Here's how the part is built. I have some questions about the finished solid (model axes, mm). Face numbers are marked on the shaded views. A direction names the side the tool comes from. Give positions to 0.01 mm unless a question says otherwise; leave off trailing zeros. Loops run counter-clockwise (first coordinate to the right, second up) from the corner with the lowest first, then second, coordinate; pieces in that order, holes last. Notation, with made-up numbers: (82.25, 9) - (98.25, 9) arc R20 ccw to (98.25, 36) - close; hole circle Ø11 at (66.25, 29). An arc over 180 degrees is marked (long way). Put each result on its own line as item: value. Start each with the question number.
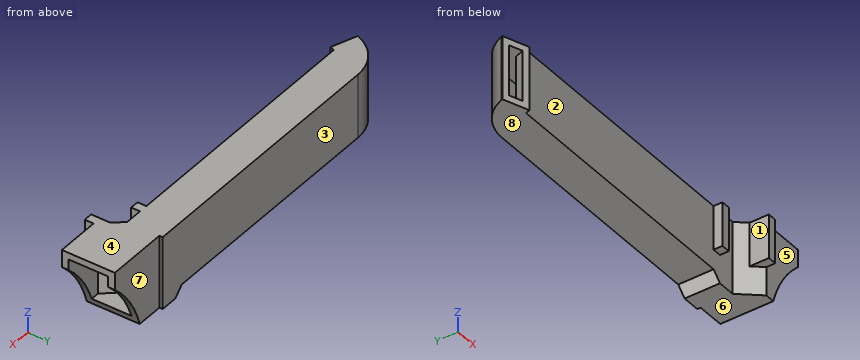
from build123d import *

# Parameters (mm, degrees)
RESSALTO_EXTRUS_O1_DEPTH = 16.5
CORTE_EXTRUS_O1_START    = -14.5
ESBO_O2_W                = 84.883298415
ESBO_O2_H                = 23.037156827
CORTE_EXTRUS_O1_DEPTH    = 14.5
CHANFRO1_SIZE            = 3
CASCA1_T                 = -1.5
CORTE_EXTRUS_O2_DEPTH    = 88.520354775
ESBO_O5_W                = 2
ESBO_O5_H                = 2
RESSALTO_EXTRUS_O2_DEPTH = 10


with BuildPart() as part:
    # Esboço1 → Ressalto-extrusão1 (new body)
    with BuildSketch(Plane.XY):
        with BuildLine():
            Line((9.53089658, 0), (71, 0))
            Line((71, 0), (71, -0.75))
            Line((71, -0.75), (85, -0.75))
            Line((85, -0.75), (85, -12.75))
            Line((85, -12.75), (75, -12.75))
            Line((75, -12.75), (71, -8))
            Line((71, -8), (6.002125959, -8))
            Line((6.002125959, -8), (5.638155725, -9))
            Line((5.638155725, -9), (0, -6.94787914))
            Line((0, -6.94787914), (0.133970372, -6.579798567))
            ThreePointArc((0.133970372, -6.579798567), (3.795132217, -1.808479557), (9.53089658, 0))
        make_face()
    extrude(amount=RESSALTO_EXTRUS_O1_DEPTH)

    # Esboço2 → Corte-extrusão1 (cut)
    with BuildSketch(Plane.XY.offset(16.5).offset(CORTE_EXTRUS_O1_START)):
        with Locations((25.558350793, -2.469824016)):
            Rectangle(ESBO_O2_W, ESBO_O2_H)
    extrude(amount=-CORTE_EXTRUS_O1_DEPTH, mode=Mode.SUBTRACT)

    # Chanfro1
    # the kernel refuses this chamfer: 3 mm, written as the material it adds along each edge
    with BuildSketch(Plane(origin=(68, 0, 2), x_dir=(-0.9996219169112968, 0, 0.027495876610586334), z_dir=(0, -1, 0))) as chanfro1_piece_1_section:
        Polygon((CHANFRO1_SIZE * 0.999621916911, CHANFRO1_SIZE * 0.0274958766106), (-CHANFRO1_SIZE * 0.0274958766106, CHANFRO1_SIZE * 0.999621916911), (0, 0), align=None)
    chanfro1_piece_1 = extrude(amount=8, mode=Mode.PRIVATE)
    chanfro1_piece_1 = split(chanfro1_piece_1, bisect_by=Plane(origin=(66.907908995, -4, 0), z_dir=(0, 0, 1)), keep=Keep.TOP, mode=Mode.PRIVATE)
    add(chanfro1_piece_1)

    # Casca1
    casca1_openings = [part.faces().sort_by_distance(p)[0] for p in [
        (85, -6.75, 8.25),
        (2.819077862, -7.97393957, 9.25),
    ]]
    offset(amount=CASCA1_T, openings=casca1_openings, kind=Kind.INTERSECTION)

    # Esboço4 → Corte-extrusão2 (cut, through all)
    with BuildSketch(Plane.XZ.offset(12.75)):
        with BuildLine():
            Line((77.16718427, 0), (85, 0))
            Line((85, 0), (85, 12.566963801))
            ThreePointArc((85, 12.566963801), (80.237763274, 6.810675399), (77.16718427, 0))
        make_face()
    extrude(amount=-CORTE_EXTRUS_O2_DEPTH, mode=Mode.SUBTRACT)

    # Esboço5 → Ressalto-extrusão2 (add)
    with BuildSketch(Plane.XY.offset(16.5)):
        with Locations((66, -9)):
            Rectangle(ESBO_O5_W, ESBO_O5_H)
        Polygon((75, -14.75), (73, -14.75), (73, -10.375), (75, -12.75), align=None)
    extrude(amount=-RESSALTO_EXTRUS_O2_DEPTH)


solid = part.part
1) I'm going to push flat-ended pins straight in: P1, Ø1, axis at x = 8.5, z = 7, coming from the +Y side; P2, Ø1.6, axis at x = 66.5, z = 11.5, coming from the -Y side; P3, Ø5, axis at x = 61, y = -5, coming from the -Z side. Where does each tip first touch, or does it pass through?
2) Suppose I cut it at C-C on y = -12. Please give me the cut outline in (x, z), plus the area to 3 significant figures.
3) Thinking about a two-plate mould opening in X: for the marked faces 1, 2 and 3, which applies, pulls with the +X half, pulls with the -X half, needs draft (parallel to the pull), parting line crosses it, or undercut?
4) Suppose I cut it at A-A on x = 11. Please give me the cut outline in (y, z), plus the area to 3 significant figures.
5) Which directions (+Z, -Z, +X, -X, +Y, -Y) give clear straight access to the entire face, cutting with the end or side of a thin tool? Please do the marked faces 4, 5, 6, 7 and 8.
6) Suppose I cut it at B-B on z = 5.5. Please give me the cut outline in (x, y).
7) I need wall thicknesses on line 1 (Y direction, x = 66.5, z = 11); line 2 (Y direction, x = 79, z = 12); line 3 (Z direction, x = 27, y = -5.5). Which ranges of each line are inside material? Lowest first, please.
Ans:
1. P1: stops at y = -0.01
1. P2: stops at y = -10
1. P3: stops at z = 2
2. outline: (73, 6.5) - (74.37, 6.5) - (74.37, 0) - (77.17, 0) arc R28 cw to (85, 12.57) - (85, 16.5) - (73, 16.5) - close
2. area: 130 mm²
3. face 1: pulls with the -X half
3. face 2: undercut
3. face 3: needs draft
4. outline: (-8, 2) - (0, 2) - (0, 16.5) - (-8, 16.5) - close; hole (-6.5, 3.5) - (-1.5, 3.5) - (-1.5, 15) - (-6.5, 15) - close
4. area: 58.5 mm²
5. face 4: +Z, +X, -X, +Y, -Y
5. face 5: +Z, -Z, +X, -Y
5. face 6: -Z, +X, -X, +Y, -Y
5. face 7: +Z, -Z, +X, +Y
5. face 8: -Z, -X, +Y, -Y
6. outline: (0, -6.95) - (1.41, -7.46) - (1.54, -7.09) arc R8.5 cw to (9.53, -1.5) - (69.5, -1.5) - (69.5, -2.25) - (79.47, -2.25) - (79.47, -0.75) - (71, -0.75) - (71, 0) - (9.53, 0) arc R10 ccw to (0.13, -6.58) - close; (4.23, -8.49) - (5.64, -9) - (6, -8) - (71, -8) - (75, -12.75) - (79.47, -12.75) - (79.47, -11.25) - (75.7, -11.25) - (71.7, -6.5) - (4.95, -6.5) - close
7. line 1: y = -10 to -6.5, -1.5 to 0
7. line 2: y = -12.75 to -11.25, -2.25 to -0.75
7. line 3: z = 2 to 3.5, 15 to 16.5
